from build123d import *

# Parameters (mm, degrees)
BOSS_EXTRUDE1_DEPTH = 2
SKETCH2_R           = 2.5
CUT_EXTRUDE1_DEPTH  = 6
SKETCH3_R           = 2.5
CUT_EXTRUDE2_DEPTH  = 6
SKETCH4_R           = 2.5
CUT_EXTRUDE3_DEPTH  = 6
SKETCH5_R           = 2.5
CUT_EXTRUDE4_DEPTH  = 6
SKETCH6_R           = 2.5
CUT_EXTRUDE5_DEPTH  = 6


with BuildPart() as part:
    # Sketch1 → Boss-Extrude1 (new body)
    with BuildSketch(Plane.XY):
        Polygon((0, 0), (62.662776372, 77.931870614), (161.485144274, 62.630249712), (98.822367902, -15.301620902), align=None)
    extrude(amount=BOSS_EXTRUDE1_DEPTH)

    # Sketch2 → Cut-Extrude1 (cut)
    with BuildSketch(Plane(origin=(0, 0, 0), x_dir=(-1, 0, 0), z_dir=(0, 0, -1))):
        with Locations((-39.124575247, 32.69965767)):
            Circle(SKETCH2_R)
    extrude(amount=-CUT_EXTRUDE1_DEPTH, mode=Mode.SUBTRACT)

    # Sketch3 → Cut-Extrude2 (cut)
    with BuildSketch(Plane(origin=(0, 0, 0), x_dir=(-1, 0, 0), z_dir=(0, 0, -1))):
        with Locations((-26.592019973, 17.113283547)):
            Circle(SKETCH3_R)
    extrude(amount=-CUT_EXTRUDE2_DEPTH, mode=Mode.SUBTRACT)

    # Sketch4 → Cut-Extrude3 (cut)
    with BuildSketch(Plane(origin=(0, 0, 0), x_dir=(-1, 0, 0), z_dir=(0, 0, -1))):
        with Locations((-130.308271813, 57.338499192)):
            Circle(SKETCH4_R)
    extrude(amount=-CUT_EXTRUDE3_DEPTH, mode=Mode.SUBTRACT)

    # Sketch5 → Cut-Extrude4 (cut)
    with BuildSketch(Plane(origin=(0, 0, 0), x_dir=(-1, 0, 0), z_dir=(0, 0, -1))):
        with Locations((-110.543798232, 60.398823373)):
            Circle(SKETCH5_R)
    extrude(amount=-CUT_EXTRUDE4_DEPTH, mode=Mode.SUBTRACT)

    # Sketch6 → Cut-Extrude5 (cut)
    with BuildSketch(Plane(origin=(0, 0, 0), x_dir=(-1, 0, 0), z_dir=(0, 0, -1))):
        with Locations((-67.776514838, 64.746663819)):
            Circle(SKETCH6_R)
    extrude(amount=-CUT_EXTRUDE5_DEPTH, mode=Mode.SUBTRACT)


solid = part.part
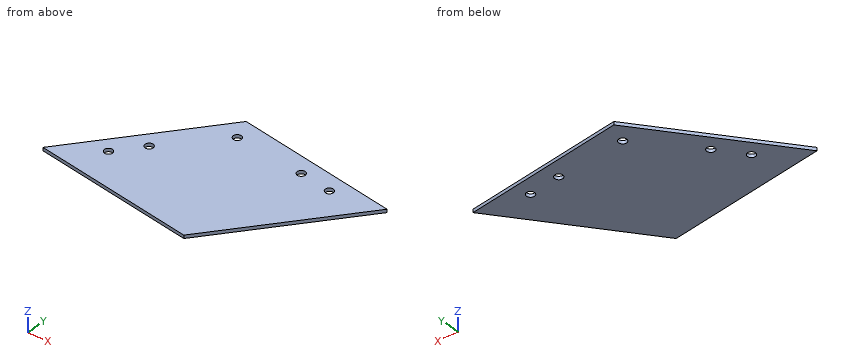
Design review of the part built by this model. Coordinates are the model's own, in mm. Coordinates: 2 decimals unless noted, no trailing zeros. Order: outer loops, then holes, each group sorted by start corner. A loop starts at its lowest first (then second) coordinate and runs counter-clockwise, first axis right, second up.
Item 1: Take a section at A-A, the plane x = 39. Write out the cut boundary in (y, z).
Item 2: For line 1 (X direction, y = 32.5, z = 1.35); line 2 (Y direction, x = 39.5, z = 0.25) (3 decimals); line 3 (X direction, y = 55.5, z = 0.35), list the stretches that pass through material, from the lowest coordinate up.
Item 3: Take a section at D-D, the plane y = -5.5. Write out the cut boundary in (x, z).
Item 4: Take a section at C-C, the plane x = 119.5. Write out the cut boundary in (y, z).
Item 5: Take a section at B-B, the plane z = 0.9. Write out the cut boundary in (x, y).
The answers:
1. outline: (-6.04, 0) - (30.2, 0) - (30.2, 2) - (-6.04, 2) - close; (35.2, 0) - (48.5, 0) - (48.5, 2) - (35.2, 2) - close
2. line 1: x = 26.13 to 36.63, 41.62 to 137.26
2. line 2: y = -6.116 to 30.228, 35.171 to 49.125
2. line 3: x = 44.63 to 128.61, 132 to 155.75
3. outline: (35.52, 0) - (106.7, 0) - (106.7, 2) - (35.52, 2) - close
4. outline: (10.41, 0) - (69.13, 0) - (69.13, 2) - (10.41, 2) - close
5. outline: (0, 0) - (98.82, -15.3) - (161.49, 62.63) - (62.66, 77.93) - close; hole circle Ø5 at (26.59, 17.11); hole circle Ø5 at (39.12, 32.7); hole circle Ø5 at (67.78, 64.75); hole circle Ø5 at (110.54, 60.4); hole circle Ø5 at (130.31, 57.34)
